from build123d import *

# Parameters (mm, degrees)
F0_R     = 10
F1_DEPTH = 20
F5_R     = 4
F6_DEPTH = 25
F7_SIZE  = 1


with BuildPart() as f1:
    # F0 (on Top) → F1 (new body)
    with BuildSketch(Plane.XY):
        Circle(F0_R)
    extrude(amount=-F1_DEPTH)

    # F2 (on Right) → F3 (revolve, cut)
    with BuildSketch(Plane.YZ):
        Polygon((10, -16), (10, -4), (5.7987547707, -10), align=None)
    revolve(axis=Axis((0, 0, 0), (0, 0, 1)), mode=Mode.SUBTRACT)

    # F5 (on face) → F6 (cut)
    with BuildSketch(Plane.XY):
        Circle(F5_R)
    extrude(amount=-F6_DEPTH, mode=Mode.SUBTRACT)

    # F7
    f7_edges = [f1.edges().sort_by_distance(p)[0] for p in [
        (-4, 0, -20),
        (-10, 0, -20),
        (-10, 0, 0),
        (-4, 0, 0),
    ]]
    chamfer(f7_edges, length=F7_SIZE)


solid = f1.part
Could you check a few things on this model? Use its own coordinates, in mm. A direction names the side the tool comes from. Round coordinates to 2 decimals unless told otherwise and drop trailing zeros. Write each loop counter-clockwise with the first axis right and the second up, starting at its lowest first coordinate (ties: lowest second). Pieces come first, ordered by that corner, then holes. Notation, with made-up numbers: (51, 7.25) - (89, 7.25) arc R23 cw to (89, 46.25) - close; hole circle Ø9 at (55.5, 24). An arc over 180 degrees is marked (long way). Put each result on its own line as item: value. Start each with the question number.
(1) I need wall thicknesses on probe 1 along Y at (x, z) = (0, -11); probe 2 along X at (y, z) = (2, -2.25); probe 3 along Y at (x, z) = (3.25, -5.25). Which ranges of each line are inside material? Lowest first, please.
(2) Will these pins go through, and if not, where does the flat tip stop? pin 1 (1 mm diameter, centred on y = -3, z = -14.5, fed in from -X); pin 2 (2 mm diameter, centred on y = 2.5, z = -14, fed in from +X); pin 3 (12 mm diameter, centred on x = 5.5, z = -6.5, fed in from +Y); pin 4 (4 mm diameter, centred on x = -1.5, z = -6, fed in from -Y).
(3) Thinking about a two-plate mould opening in X: for faces 3 (the cylindrical face through (9.54, 3, -2.48)), 4 (the cylindrical face through (-0.867, -3.905, -9.874)), 5 (the flat face through (4, -4, 0)), which applies, released by +X, released by -X, zero draft, split by the parting line, or undercut?
(4) I want a section at A-A, the plane y = 0. Please give me the cut outline in (x, z), plus the area to 3 significant figures.
(5) I want a section at C-C, the plane z = -16.75. Please give me the cut outline in (x, y), plus the area to 3 significant figures.
(6) I want a section at D-D, the plane z = -11.5. Please give me the cut outline in (x, y).
(7) For faces 1 (the cylindrical face through (9.54, 3, -17.48)), 2 (the conical face through (5.86, -1.3, -9.71)), which set-ups out of +Z, -Z, +X, -X, +Y, -Y let a thin tool reach every point of the face, with its end or its side?
Here are the results:
1. probe 1: y = -6.5 to -4, 4 to 6.5
1. probe 2: x = -9.8 to -3.46, 3.46 to 9.8
1. probe 3: y = -8.53 to -2.33, 2.33 to 8.53
2. pin 1: stops at x = -8.84
2. pin 2: stops at x = 9
2. pin 3: stops at y = 10
2. pin 4: stops at y = -9.91
3. face 3: split by the parting line
3. face 4: undercut
3. face 5: zero draft
4. outline: (-10, -19) - (-9, -20) - (-5, -20) - (-4, -19) - (-4, -1) - (-5, 0) - (-9, 0) - (-10, -1) - (-10, -4) - (-5.8, -10) - (-10, -16) - close; (4, -19) - (5, -20) - (9, -20) - (10, -19) - (10, -16) - (5.8, -10) - (10, -4) - (10, -1) - (9, 0) - (5, 0) - (4, -1) - close
4. area: 186 mm^2
5. outline: circle Ø20 at (0, 0); hole circle Ø8 at (0, 0)
5. area: 264 mm^2
6. outline: circle Ø13.7 at (0, 0); hole circle Ø8 at (0, 0)
7. face 1: +Z, -Z
7. face 2: none
